Part model, mm, in its own coordinate system. Coordinates: 2 decimals unless noted, no trailing zeros. Order: outer loops, then holes, each group sorted by start corner. A loop starts at its lowest first (then second) coordinate and runs counter-clockwise, first axis right, second up.
from build123d import *


with BuildPart() as part:
    # Sketch1 → Revolve1 (revolve)
    with BuildSketch(Plane(origin=(0, 0, 0), x_dir=(-1, 0, 0), z_dir=(0, 0, -1))):
        with BuildLine():
            Line((-6, -21), (-6, -5))
            Line((-6, -5), (-2.5, -5))
            Line((-2.5, -5), (-2.5, 0))
            Line((-2.5, 0), (-9, 0))
            ThreePointArc((-9, 0), (-9.707106781, -0.292893219), (-10, -1))
            Line((-10, -1), (-10, -21))
            ThreePointArc((-10, -21), (-9.707106781, -21.707106781), (-9, -22))
            Line((-9, -22), (-7, -22))
            ThreePointArc((-7, -22), (-6.292893219, -21.707106781), (-6, -21))
        make_face()
    revolve(axis=Axis((0, -22, 0), (0, 1, 0)))


solid = part.part
Q1. Cut at C-C on y = -2.5. Write the cut outline in (x, z), and give its area (3 significant figures).
Results list:
outline: circle Ø20 at (0, 0); hole circle Ø5 at (0, 0)
area: 295 mm2
Q2. Mould opens along Z. For faces 1 (the face through (3, -5, 0)), 2 (the face through (-6, -13, 0)), 3 (the face through (-2.17, -11.14, 9.76)), 4 (the face through (-2, 0, 2)) say: pulls with the +Z half, pulls with the -Z half, needs draft (parallel to the pull), parting line crosses it, or undercut.
Results list:
face 1: undercut
face 2: undercut
face 3: parting line crosses it
face 4: needs draft
Q3. Pin check, flat tips, straight feed: pin 1 Ø1.5 at (y, z) = (-2.5, 1) entering from +X; pin 2 Ø1.5 at (y, z) = (-13, 6.5) entering from +X; pin 3 Ø6 at (x, y) = (-5, -14) entering from +Z. Stop position of each tip, or through.
Results list:
pin 1: stops at x = 10
pin 2: stops at x = 8.18
pin 3: stops at z = 9.8
Q4. Cut at A-A on z = 0. Write the cut outline in (x, y).
Results list:
outline: (-10, -21) arc R1 ccw to (-9, -22) - (-7, -22) arc R1 ccw to (-6, -21) - (-6, -5) - (-2.5, -5) - (-2.5, 0) - (-9, 0) arc R1 ccw to (-10, -1) - close; (2.5, -5) - (6, -5) - (6, -21) arc R1 ccw to (7, -22) - (9, -22) arc R1 ccw to (10, -21) - (10, -1) arc R1 ccw to (9, 0) - (2.5, 0) - close
Q5. Cut at D-D on y = -18.25. Write the cut outline in (x, z).
Results list:
outline: circle Ø20 at (0, 0); hole circle Ø12 at (0, 0)
Q6. Wall check: line 1 along Z through (x, y) = (0, -14.25); line 2 along X through (y, z) = (-3.05, 0). Give the ranges that are in metal, low to high.
Results list:
line 1: z = -10 to -6, 6 to 10
line 2: x = -10 to -2.5, 2.5 to 10
Q7. Cut at B-B on x = 0. Write the cut outline in (y, z).
Results list:
outline: (-22, -9) arc R1 ccw to (-21, -10) - (-1, -10) arc R1 ccw to (0, -9) - (0, -2.5) - (-5, -2.5) - (-5, -6) - (-21, -6) arc R1 ccw to (-22, -7) - close; (-22, 7) arc R1 ccw to (-21, 6) - (-5, 6) - (-5, 2.5) - (0, 2.5) - (0, 9) arc R1 ccw to (-1, 10) - (-21, 10) arc R1 ccw to (-22, 9) - close
